Design review of the part built by this model. Coordinates are the model's own, in mm. Round coordinates to 2 decimals unless told otherwise and drop trailing zeros. Loops run counter-clockwise (first coordinate to the right, second up) from the corner with the lowest first, then second, coordinate; pieces in that order, holes last. Notation, with made-up numbers: M 50.5,69.25 L 91.5,69.25 A23 ccw 91.5,91.25 Z; hole C -24.5,70.25 d3. An arc over 180 degrees is marked long. Use a Markdown table: item, result.
from build123d import *

# Parameters (mm, degrees)
SKETCH_1_R      = 1
SKETCH_1_R_2    = 1.5
EXTRUDE_1_DEPTH = 2


with BuildPart() as part:
    # 草图1 → 凸台-拉伸1 (new body)
    with BuildSketch(Plane(origin=(0, 0, 0), x_dir=(0, 0, -1), z_dir=(1, 0, 0))):
        with BuildLine():
            Line((107.863715966, -104.404074838), (101.845843381, -108.686473232))
            ThreePointArc((101.845843381, -108.686473232), (100.236001316, -109.005608731), (98.929340159, -108.012595355))
            ThreePointArc((98.929340159, -108.012595355), (95.996901234, -102.756809465), (92.952174798, -97.565265927))
            ThreePointArc((92.952174798, -97.565265927), (92.67119221, -96.396525563), (93.110928625, -95.277804356))
            ThreePointArc((93.110928625, -95.277804356), (93.386262354, -90.634283432), (89.082079375, -88.870167754))
            ThreePointArc((89.082079375, -88.870167754), (87.883298953, -88.781676215), (86.951761021, -88.02197737))
            ThreePointArc((86.951761021, -88.02197737), (63.249240179, -56.927091802), (35.446375502, -29.437055089))
            ThreePointArc((35.446375502, -29.437055089), (34.93756912, -29.118601809), (34.357184804, -28.965466337))
            ThreePointArc((34.357184804, -28.965466337), (31.162596189, -27.612410648), (29.250996223, -24.717252331))
            ThreePointArc((29.250996223, -24.717252331), (28.99483955, -24.174407799), (28.589143834, -23.732019493))
            ThreePointArc((28.589143834, -23.732019493), (13.863721442, -12.651321704), (-1.558710581, -2.56328331))
            ThreePointArc((-1.558710581, -2.56328331), (-2.635591887, 1.433058061), (1.304059018, 2.701745746))
            ThreePointArc((1.304059018, 2.701745746), (18.225711529, -6.316411442), (34.373430157, -16.656656404))
            ThreePointArc((34.373430157, -16.656656404), (34.856722013, -16.904193707), (35.388785697, -17.012609443))
            ThreePointArc((35.388785697, -17.012609443), (38.521022393, -18.141769735), (40.568988637, -20.766982858))
            ThreePointArc((40.568988637, -20.766982858), (40.837621253, -21.238875062), (41.223285286, -21.621117118))
            ThreePointArc((41.223285286, -21.621117118), (79.319293236, -57.386189934), (108.771734361, -100.548673263))
            ThreePointArc((108.771734361, -100.548673263), (109.044434758, -102.647527604), (107.863715966, -104.404074838))
        make_face()
        with Locations((100.83272848, -103.814691777)):
            Circle(SKETCH_1_R, mode=Mode.SUBTRACT)
        with Locations((104.83272848, -100.814691777)):
            Circle(SKETCH_1_R, mode=Mode.SUBTRACT)
        with Locations((35, -23)):
            Circle(SKETCH_1_R_2, mode=Mode.SUBTRACT)
        Circle(SKETCH_1_R_2, mode=Mode.SUBTRACT)
    extrude(amount=EXTRUDE_1_DEPTH)


solid = part.part
1. The part is to be moulded in two halves that separate along Y. For faces 1 (the face through (0.986, 1.377, 2.666)), 2 (the face through (0.99, 0.07, 1.5)), 3 (the face through (0.99, -18.11, -38.48)), 4 (the face through (0.986, -27.644, -31.201)), say which applies: pulls with the +Y half, pulls with the -Y half, needs draft (parallel to the pull), parting line crosses it, or undercut.
Check values:
| item | result |
|---|---|
| face 1 | parting line crosses it |
| face 2 | undercut |
| face 3 | pulls with the +Y half |
| face 4 | pulls with the -Y half |
2. Take a section at D-D on y = -51. Give the boundary of the cut face in (x, z).
Check values:
| item | result |
|---|---|
| outline | M 0,-73.65 L 2,-73.65 L 2,-57.89 L 0,-57.89 Z |
3. Wall thickness on line 1 along Z through (x, y) = (0.7, -22.5); line 2 along Y through (x, z) = (0.7, 0); line 3 along Y through (x, z) = (1.3, -34): over which ranges is each line inside the solid? List them lowest first. Write a range as from..to.
Check values:
| item | result |
|---|---|
| line 1 | z = -42.38..-36.41, -33.59..-27.05 |
| line 2 | y = -3.52..-1.5, 1.5..3 |
| line 3 | y = -28.92..-24.12, -21.88..-16.4 |
4. Take a section at A-A on z = 0. Give the boundary of the cut face in (x, y), and give its area (3 significant figures).
Check values:
| item | result |
|---|---|
| outline | M 0,-3.52 L 2,-3.52 L 2,-1.5 L 0,-1.5 Z; M 0,1.5 L 2,1.5 L 2,3 L 0,3 Z |
| area | 7.04 mm² |
5. Insertion check: pin 1 (1 mm diameter, centred on x = 0.5, z = -17, fed in from -Y). The pin has a flat end and moves straight along its axis. Give the tip position at first contact, or say it passes through.
Check values:
| item | result |
|---|---|
| pin 1 | stops at y = -15.25 |
6. Take a section at C-C on x = 1.25. Give the boundary of the cut face in (y, z) (3 decimals).
Check values:
| item | result |
|---|---|
| outline | M -108.686,-101.846 L -104.404,-107.864 A3 ccw -100.549,-108.772 A240 ccw -21.621,-41.223 A2 cw -20.767,-40.569 A6 ccw -17.013,-35.389 A2 cw -16.657,-34.373 A240 ccw 2.702,-1.304 A3 ccw -2.563,1.559 A280 cw -23.732,-28.589 A2 cw -24.717,-29.251 A6 ccw -28.965,-34.357 A2 cw -29.437,-35.446 A280 cw -88.022,-86.952 A2 ccw -88.87,-89.082 A4 cw -95.278,-93.111 A2 ccw -97.565,-92.952 A280 cw -108.013,-98.929 A2 ccw Z; hole C -103.815,-100.833 d2; hole C -100.815,-104.833 d2; hole C -23,-35 d3; hole C 0,0 d3 |
7. Take a section at B-B on y = 0. Give the boundary of the cut face in (x, z).
Check values:
| item | result |
|---|---|
| outline | M 0,-6.73 L 2,-6.73 L 2,-1.5 L 0,-1.5 Z; M 0,1.5 L 2,1.5 L 2,3 L 0,3 Z |
